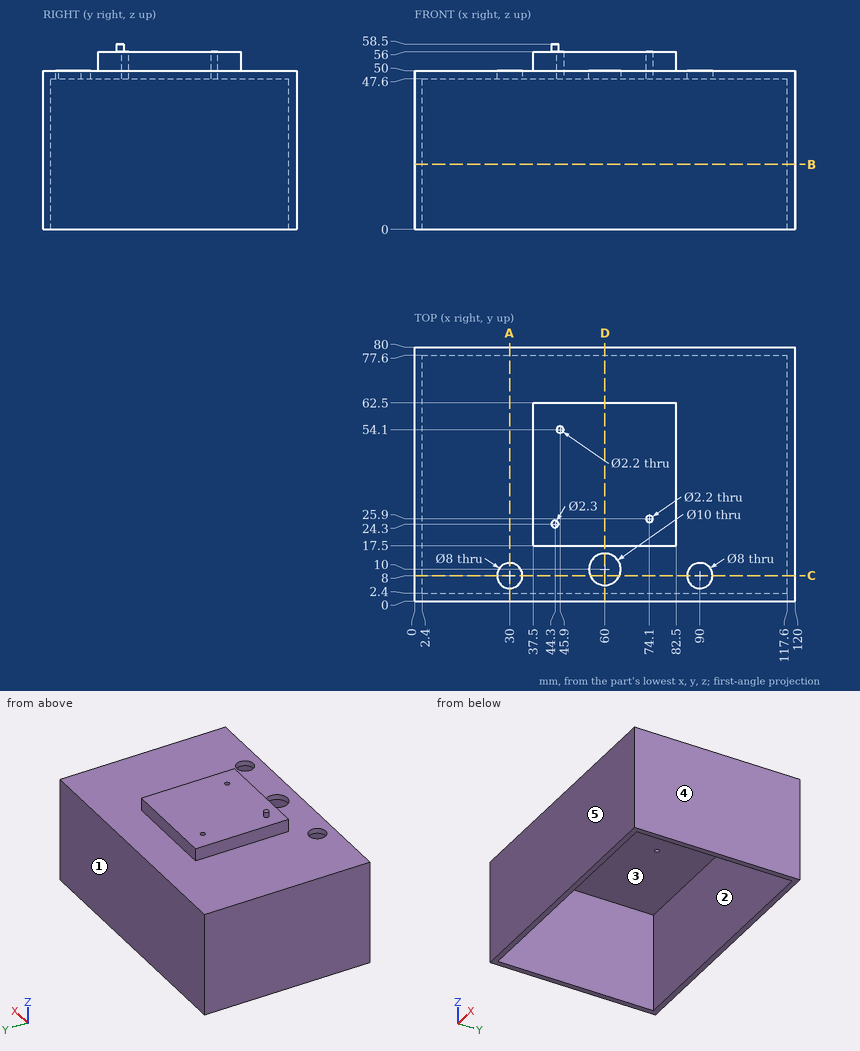
Design review of the part shown in the three views and the two pictorial views. Dimensions are in mm from the part's minimum x, y and z. A direction names the side the tool comes from. Round coordinates to 2 decimals unless told otherwise and drop trailing zeros. Write each loop counter-clockwise with the first axis right and the second up, starting at its lowest first coordinate (ties: lowest second). Pieces come first, ordered by that corner, then holes. Notation, with made-up numbers: (75.25, -37.5) - (125.25, -37.5) arc R16 ccw to (125.25, -17.5) - close; hole circle Ø5 at (11, 69.5). An arc over 180 degrees is marked (long way). Return JSON: item names as keys, results as strings. Group by question number.
Item 1: We need section B-B on z = 20.5. Write out the cut boundary in (x, y), and give its area (3 significant figures).
Item 2: Insertion check: P1, Ø3.5, axis at x = 45.9, y = 54.1, coming from the -Z side; P2, Ø1, axis at x = 46, y = 25, coming from the +Z side; P3, Ø3, axis at x = 68, z = 52, coming from the -Y side. Each pin has a flat end and moves straight along its axis. Give the tip position at first contact, or say it passes through.
Item 3: The part is to be moulded in two halves that separate along Y. For the marked faces 3, 4 and 5, say which applies: pulls with the +Y half, pulls with the -Y half, needs draft (parallel to the pull), parting line crosses it, or undercut.
Item 4: Machinability: for the marked faces 1 and 2, which of the approach directions +Z, -Z, +X, -X, +Y, -Y give a long, thin tool a straight path to every point of the face, cutting with its end or side? Answer none if there is none.
Item 5: We need section A-A on x = 30. Write out the cut boundary in (y, z).
Item 6: We need section D-D on x = 60. Write out the cut boundary in (y, z).
Item 7: We need section C-C on y = 8. Write out the cut boundary in (x, z), and give its area (3 significant figures).
Item 8: For probe 1 along Y at (x, z) = (110, 26); probe 2 along Y at (x, z) = (45.9, 49.5); probe 3 along X at (y, z) = (71, 7.5), list the stretches that pass through material, from the lowest coordinate up. Write a range as [from, to].
Model answer:
{
 "1": {"outline": "(0, 0) - (120, 0) - (120, 80) - (0, 80) - close; hole (2.4, 2.4) - (117.6, 2.4) - (117.6, 77.6) - (2.4, 77.6) - close", "area": "937 mm²"},
 "2": {"P1": "stops at z = 47.6", "P2": "stops at z = 56", "P3": "stops at y = 17.5"},
 "3": {"face 3": "undercut", "face 4": "needs draft", "face 5": "pulls with the -Y half"},
 "4": {"face 1": "+Z, -Z, +X, -X, +Y", "face 2": "-Z"},
 "5": {"outline": "(0, 0) - (2.4, 0) - (2.4, 47.6) - (4, 47.6) - (4, 50) - (0, 50) - close; (12, 47.6) - (77.6, 47.6) - (77.6, 0) - (80, 0) - (80, 50) - (12, 50) - close"},
 "6": {"outline": "(0, 0) - (2.4, 0) - (2.4, 47.6) - (5, 47.6) - (5, 50) - (0, 50) - close; (15, 47.6) - (77.6, 47.6) - (77.6, 0) - (80, 0) - (80, 50) - (62.5, 50) - (62.5, 56) - (17.5, 56) - (17.5, 50) - (15, 50) - close"},
 "7": {"outline": "(0, 0) - (2.4, 0) - (2.4, 47.6) - (26, 47.6) - (26, 50) - (0, 50) - close; (34, 47.6) - (55.42, 47.6) - (55.42, 50) - (34, 50) - close; (64.58, 47.6) - (86, 47.6) - (86, 50) - (64.58, 50) - close; (94, 47.6) - (117.6, 47.6) - (117.6, 0) - (120, 0) - (120, 50) - (94, 50) - close", "area": "456 mm²"},
 "8": {"probe 1": "y = [0, 2.4], [77.6, 80]", "probe 2": "y = [0, 53], [55.2, 80]", "probe 3": "x = [0, 2.4], [117.6, 120]"}
}
